Geometry: final body of the model. Coordinates: model frame, mm. Face numbers are marked on the shaded views. A direction names the side the tool comes from. Give positions to 0.01 mm unless a question says otherwise; leave off trailing zeros. Write each loop counter-clockwise with the first axis right and the second up, starting at its lowest first coordinate (ties: lowest second). Pieces come first, ordered by that corner, then holes.
from build123d import *

# Parameters (mm, degrees)
SKETCH1_W           = 20
SKETCH1_H           = 20
BOSS_EXTRUDE1_DEPTH = 30
FILLET1_R           = 1
SKETCH2_R           = 8
BOSS_EXTRUDE2_DEPTH = 1.8
SKETCH3_R           = 2
BOSS_EXTRUDE3_DEPTH = 8.2
SKETCH4_R           = 1
CUT_EXTRUDE1_DEPTH  = 3


with BuildPart() as part:
    # Sketch1 → Boss-Extrude1 (new body)
    with BuildSketch(Plane.XY):
        Rectangle(SKETCH1_W, SKETCH1_H)
    extrude(amount=BOSS_EXTRUDE1_DEPTH)

    # Fillet1
    fillet1_edges = [part.edges().sort_by_distance(p)[0] for p in [
        (10, -10, 15),
        (-10, -10, 15),
        (-10, 10, 15),
        (10, 10, 15),
    ]]
    fillet(fillet1_edges, radius=FILLET1_R)

    # Sketch2 → Boss-Extrude2 (add)
    with BuildSketch(Plane.XY.offset(30)):
        Circle(SKETCH2_R)
    extrude(amount=BOSS_EXTRUDE2_DEPTH)

    # Sketch3 → Boss-Extrude3 (add)
    with BuildSketch(Plane.XY.offset(31.8)):
        Circle(SKETCH3_R)
    extrude(amount=BOSS_EXTRUDE3_DEPTH)

    # Sketch4 → Cut-Extrude1 (cut)
    with BuildSketch(Plane.XY.offset(30)):
        with Locations((-7.7, 7.7)):
            Circle(SKETCH4_R)
        with Locations((7.7, 7.7)):
            Circle(SKETCH4_R)
        with Locations((7.7, -7.7)):
            Circle(SKETCH4_R)
        with Locations((-7.7, -7.7)):
            Circle(SKETCH4_R)
    extrude(amount=-CUT_EXTRUDE1_DEPTH, mode=Mode.SUBTRACT)


solid = part.part
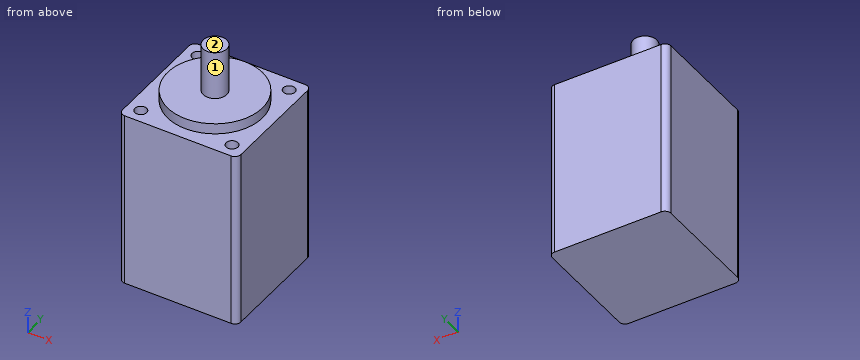
Q1. Section A-A on x = 0. Output: boundary loops of the cut face in (y, z).
Filled sheet:
outline: (-10, 0) - (10, 0) - (10, 30) - (8, 30) - (8, 31.8) - (2, 31.8) - (2, 40) - (-2, 40) - (-2, 31.8) - (-8, 31.8) - (-8, 30) - (-10, 30) - close
Q2. Ray query, line 1 along Y through (x, z) = (7.7, 28.3); line 2 along Z through (x, y) = (-5.5, 1.75); line 3 along Z through (x, y) = (6.5, -8.5). Return the intervals inside material, ascending.
Filled sheet:
line 1: y = -10 to -8.7, -6.7 to 6.7, 8.7 to 10
line 2: z = 0 to 31.8
line 3: z = 0 to 30
Q3. Pin query (flat end, axial travel): P1, Ø6, axis at x = 7, y = 6.5, coming from the -Z side; P2, Ø2, axis at x = -8, y = 8, coming from the +Z side; P3, Ø1.6, axis at x = 7.7, y = 7.7, coming from the +Z side; P4, Ø5, axis at x = 7.5, y = 7, coming from the +Z side. Return the tip coordinate at first contact, or that it passes through.
Filled sheet:
P1: stops at z = 0
P2: stops at z = 30
P3: stops at z = 27
P4: stops at z = 31.8
Q4. Section C-C on x = 4. Output: boundary loops of the cut face in (y, z).
Filled sheet:
outline: (-10, 0) - (10, 0) - (10, 30) - (6.93, 30) - (6.93, 31.8) - (-6.93, 31.8) - (-6.93, 30) - (-10, 30) - close
Q5. Access query for the marked faces 1 and 2. Directions: +Z, -Z, +X, -X, +Y, -Y. A direction counts if a zero-diameter tool reaches every point of the face in a straight line with its end or side. Return the directions, or none.
Filled sheet:
face 1: +Z
face 2: +Z, +X, -X, +Y, -Y
